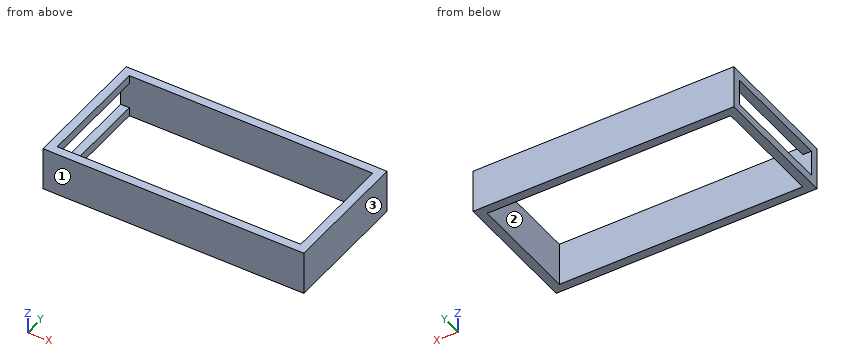
from build123d import *

# Parameters (mm, degrees)
F0_W     = 150
F0_H     = 75
F1_DEPTH = 25
F2_T     = -5
F3_W     = 140
F3_H     = 65
F4_DEPTH = 25.001


with BuildPart() as f1:
    # F0 (on Top) → F1 (new body)
    with BuildSketch(Plane.XY):
        Rectangle(F0_W, F0_H)
    extrude(amount=F1_DEPTH)

    # F2
    f2_openings = [f1.faces().sort_by_distance(p)[0] for p in [
        (-75, 0, 12.5),
    ]]
    offset(amount=F2_T, openings=f2_openings)

    # F3 (on Top) → F4 (cut, through all)
    with BuildSketch(Plane.XY):
        Rectangle(F3_W, F3_H)
    extrude(amount=F4_DEPTH, mode=Mode.SUBTRACT)


solid = f1.part
Work out the finished part from the listing and answer in its coordinate system (mm). Face numbers are marked on the shaded views. Give positions to 0.01 mm unless a question says otherwise; leave off trailing zeros. Write each loop counter-clockwise with the first axis right and the second up, starting at its lowest first coordinate (ties: lowest second). Pieces come first, ordered by that corner, then holes.
Q1. Given pin 1 (4 mm diameter, centred on x = -73, y = 3.5, fed in from -Z); pin 2 (1 mm diameter, centred on y = -13, z = 17, fed in from -X), each flat-ended and moving along its own axis, determine where each tip first touches the part or whether it passes through.
Answer:
pin 1: stops at z = 0
pin 2: stops at x = 70
Q2. Straight lines are drawn through the part: L1, parallel to Y at x = -14, z = 17.75; L2, parallel to X at y = 28.5, z = 1; L3, parallel to X at y = -29.5, z = 11.25. For each, find the intervals that lie inside material, in ascending order.
Answer:
L1: y = -37.5 to -32.5, 32.5 to 37.5
L2: x = -75 to -70, 70 to 75
L3: x = 70 to 75
Q3. The part is cut by section B-B on y = 7. Give the vertices of the cut face in (x, z), and give its area (3 significant figures).
Answer:
outline: (-75, 0) - (-70, 0) - (-70, 5) - (-75, 5) - close; (-75, 20) - (-70, 20) - (-70, 25) - (-75, 25) - close; (70, 0) - (75, 0) - (75, 25) - (70, 25) - close
area: 175 mm2
Q4. The part is cut by section C-C on z = 17.75. Give the vertices of the cut face in (x, y).
Answer:
outline: (-75, -37.5) - (75, -37.5) - (75, 37.5) - (-75, 37.5) - (-75, 32.5) - (70, 32.5) - (70, -32.5) - (-75, -32.5) - close
Q5. The part is cut by section A-A on x = -32. Give the vertices of the cut face in (y, z).
Answer:
outline: (-37.5, 0) - (-32.5, 0) - (-32.5, 25) - (-37.5, 25) - close; (32.5, 0) - (37.5, 0) - (37.5, 25) - (32.5, 25) - close
Q6. For a pull along X with two mould halves and no side action, classify the marked faces 1, 2 and 3 as released by +X, released by -X, zero draft, split by the parting line, or undercut.
Answer:
face 1: zero draft
face 2: undercut
face 3: released by +X
